Input: part model. Units: mm. Frame: model coordinates. Coordinates: 2 decimals unless noted, no trailing zeros. Order: outer loops, then holes, each group sorted by start corner. A loop starts at its lowest first (then second) coordinate and runs counter-clockwise, first axis right, second up. Notation, with made-up numbers: M 63,78 L 86,78 A19 cw 86,108 Z; hole C -14,2 d8. An arc over 180 degrees is marked long. Answer in a Markdown table with one row per item.
from build123d import *

# Parameters (mm, degrees)
SKETCH1_R           = 8.382
SKETCH1_R_2         = 6.35
BOSS_EXTRUDE1_DEPTH = 228.6
CUT_EXTRUDE1_DEPTH  = 228.6


with BuildPart() as part:
    # Sketch1 → Boss-Extrude1 (new body)
    with BuildSketch(Plane(origin=(0, 0, 0), x_dir=(1, 0, 0), z_dir=(0, 1, 0))):
        with Locations(Location((0, 0, 0), (0, 0, 270))):
            Circle(SKETCH1_R)
        with Locations(Location((0, 0, 0), (0, 0, 270))):
            Circle(SKETCH1_R_2, mode=Mode.SUBTRACT)
    extrude(amount=BOSS_EXTRUDE1_DEPTH)

    # Sketch3 → Cut-Extrude1 (cut)
    with BuildSketch(Plane(origin=(0, 0, 0), x_dir=(0, 0, -1), z_dir=(1, 0, 0))):
        with BuildLine():
            Line((-2.417681697, -8.09513592), (-2.417681697, 43.280600145))
            ThreePointArc((-2.417681697, 43.280600145), (0, 45.698281842), (2.417681697, 43.280600145))
            Line((2.417681697, 43.280600145), (2.417681697, -8.09513592))
            ThreePointArc((2.417681697, -8.09513592), (0, -10.512817617), (-2.417681697, -8.09513592))
        make_face()
    extrude(amount=-CUT_EXTRUDE1_DEPTH, mode=Mode.SUBTRACT)


solid = part.part
1) Contact query for flat-ended pins moving along their axis: pin 1 (1.1 mm diameter, centred on x = -6.5, y = 21.5, fed in from +Z); pin 2 (1.1 mm diameter, centred on x = -7.5, y = 15.5, fed in from -Z); pin 3 (5 mm diameter, centred on y = 151, z = -6, fed in from -X). Output: stop coordinate, or through.
Resolved:
| item | result |
|---|---|
| pin 1 | stops at z = 5.9 |
| pin 2 | stops at z = -4.69 |
| pin 3 | stops at x = -7.62 |
2) Mould query, pull axis X, two halves, no side actions, for faces 1 (the face through (6, 228.6, 3)), 2 (the face through (7.068, 112.7, 4.506)), 3 (the face through (6.3, 112.7, -0.8)). Classes: +X half, -X half, draft (parallel to the pull), parting line (faces both ways), or undercut.
Resolved:
| item | result |
|---|---|
| face 1 | draft |
| face 2 | parting line |
| face 3 | undercut |
3) Cut plane C-C, the plane y = 65.5. Output: boundary loops of the cut face in (x, z).
Resolved:
| item | result |
|---|---|
| outline | C 0,0 d16.76; hole C 0,0 d12.7 |
4) Cut plane B-B, the plane z = 0. Output: boundary loops of the cut face in (x, y).
Resolved:
| item | result |
|---|---|
| outline | M -8.38,45.7 L -6.35,45.7 L -6.35,228.6 L -8.38,228.6 Z; M 6.35,0 L 8.38,0 L 8.38,228.6 L 6.35,228.6 Z |
5) Material intervals for probe 1 along Z at (x, y) = (0, 108); probe 2 along X at (y, z) = (190.5, -1.25), sorted ascending.
Resolved:
| item | result |
|---|---|
| probe 1 | z = -8.38 to -6.35, 6.35 to 8.38 |
| probe 2 | x = -8.29 to -6.23, 6.23 to 8.29 |
6) Cut plane A-A, the plane x = 0. Output: boundary loops of the cut face in (y, z).
Resolved:
| item | result |
|---|---|
| outline | M 0,-8.38 L 228.6,-8.38 L 228.6,-6.35 L 0,-6.35 Z; M 0,6.35 L 228.6,6.35 L 228.6,8.38 L 0,8.38 Z |
